```python
from build123d import *


with BuildPart() as f1:
    # F0 (on Front) → F1 (revolve)
    with BuildSketch(Plane.XZ):
        with BuildLine():
            Line((-67.176946, 0), (0, 0))
            Line((0, 0), (52.278299, 0))
            Line((52.278299, 0), (52.278299, 15.29772))
            Line((52.278299, 15.29772), (22.426098, 15.29772))
            ThreePointArc((22.426098, 15.29772), (18.890564, 16.762186), (17.426098, 20.29772))
            Line((17.426098, 20.29772), (17.426098, 23.27914))
            Line((17.426098, 23.27914), (-21.682857, 23.27914))
            Line((-21.682857, 23.27914), (-21.682857, 17.105153))
            ThreePointArc((-21.682857, 17.105153), (-23.147323, 13.569619), (-26.682857, 12.105153))
            Line((-26.682857, 12.105153), (-67.176946, 12.105153))
            Line((-67.176946, 12.105153), (-67.176946, 0))
        make_face()
    revolve(axis=Axis((-33.588473, 0, 0), (-1, 0, 0)))


solid = f1.part
```
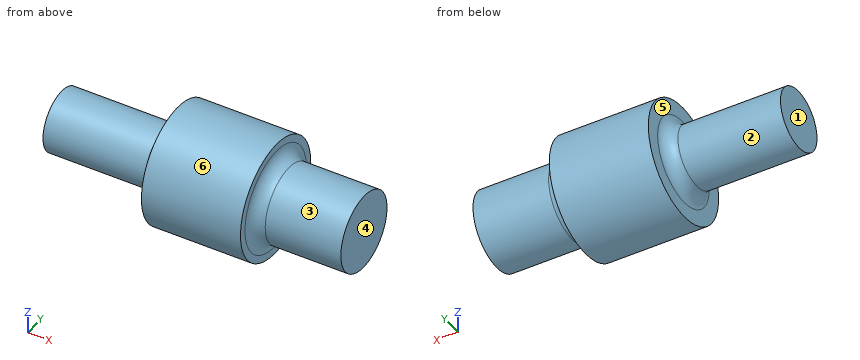
Verification items for the finished model (mm, model axes). Face numbers are marked on the shaded views. A direction names the side the tool comes from. Give positions to 0.01 mm unless a question says otherwise; leave off trailing zeros. Loops run counter-clockwise (first coordinate to the right, second up) from the corner with the lowest first, then second, coordinate; pieces in that order, holes last.
1. Mould release check, pull along X, two halves, no side actions. Record for the marked faces 4, 5 and 6: released by +X, released by -X, zero draft, split by the parting line, or undercut.
2. Section check A-A, the plane z = 0. Enter the section's corners in (x, y).
3. Go/stop test with flat-tipped pins: pin 1 Ø5 at (x, y) = (-24.5, 17) entering from -Z; pin 2 Ø10 at (x, y) = (-48.5, -6) entering from +Z; pin 3 Ø4 at (x, z) = (-21.5, 5.5) entering from +Y; pin 4 Ø1 at (x, y) = (-2.5, -11.5) entering from -Z. Record where each tip stops, or that it passes through.
4. Section check C-C, the plane x = -10. Enter the section's corners in (y, z).
5. Set-up check for the marked faces 1, 2 and 3: record each of +Z, -Z, +X, -X, +Y, -Y from which the full face is reachable in a straight line by a thin tool's end or side.
6. Section check D-D, the plane x = -53.5. Enter the section's corners in (y, z).
7. Thickness scan on line 1 (X direction, y = 14.5, z = -14); line 2 (X direction, y = 12.5, z = 0); line 3 (Y direction, x = 43.5, z = -1.5). Record the ranges inside material, lowest first.
Geometry says:
1. face 4: released by +X
1. face 5: released by -X
1. face 6: zero draft
2. outline: (-67.18, -12.11) - (-26.68, -12.11) arc R5 cw to (-21.68, -17.11) - (-21.68, -23.28) - (17.43, -23.28) - (17.43, -20.3) arc R5 cw to (22.43, -15.3) - (52.28, -15.3) - (52.28, 15.3) - (22.43, 15.3) arc R5 cw to (17.43, 20.3) - (17.43, 23.28) - (-21.68, 23.28) - (-21.68, 17.11) arc R5 cw to (-26.68, 12.11) - (-67.18, 12.11) - close
3. pin 1: passes through
3. pin 2: stops at z = 12.06
3. pin 3: stops at y = 23.01
3. pin 4: stops at z = -20.52
4. outline: circle Ø46.56 at (0, 0)
5. face 1: +Z, -Z, -X, +Y, -Y
5. face 2: -X
5. face 3: +X
6. outline: circle Ø24.21 at (0, 0)
7. line 1: x = -21.68 to 17.43
7. line 2: x = -24.74 to 52.28
7. line 3: y = -15.22 to 15.22
